Input: dimensioned drawing with shaded views. Units: mm. Origin: part minimum x, y, z. A direction names the side the tool comes from. Round coordinates to 2 decimals unless told otherwise and drop trailing zeros. Order: outer loops, then holes, each group sorted by start corner. A loop starts at its lowest first (then second) coordinate and runs counter-clockwise, first axis right, second up. Notation, with made-up numbers: M -30,1 L 5,1 A21 ccw 5,31 Z; hole C 4,8.5 d9. An arc over 180 degrees is marked long. Use one line per item in the form item = value. Start each with the question number.
Q1. Contact query for flat-ended pins moving along their axis: pin 1 (9 mm diameter, centred on x = 22, z = 10, fed in from +Y); pin 2 (1 mm diameter, centred on x = 29, z = 6, fed in from -Y); pin 3 (1.2 mm diameter, centred on x = 14, y = 1, fed in from -Z). Output: stop coordinate, or through.
Q2. Reachability of the marked faces 4, 5 and 6 from +Z, -Z, +X, -X, +Y, -Y: full face, straight path, thin tool, end or side. Return the list, or none.
Q3. Section C-C (z = 3.75). Return the cut outline in (x, y), plus the area to 3 significant figures.
Q4. Section D-D (x = 9.5). Return the cut outline in (y, z).
Q5. Pull-direction query (X, two-part tool) for the marked faces 1, 2 and 3; classes: pulls with the +X half, pulls with the -X half, needs draft (parallel to the pull), parting line crosses it, or undercut.
Q6. Section B-B (x = 22). Return the cut outline in (y, z).
Q7. Material intervals for probe 1 along X at (y, z) = (21.75, 10); probe 2 along X at (y, z) = (4.05, 10); probe 3 along Y at (x, z) = (31, 2), sorted ascending.
Q8. Section A-A (y = 14.5). Return the cut outline in (x, z).
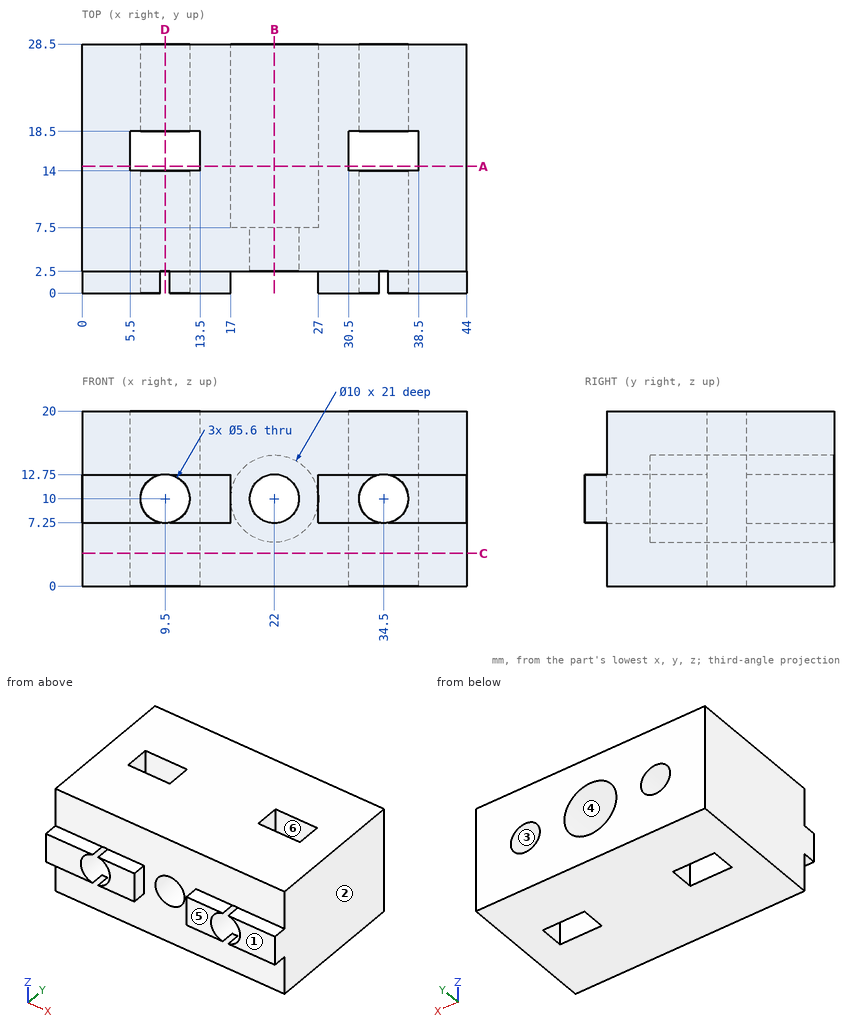
Results list:
q1.pin_1 = 7.5
q1.pin_2 = 2.5
q1.pin_3 = 7.25
q2.face_4 = +Y
q2.face_5 = +Z, -Z, +X, -X, -Y
q2.face_6 = +Z, -Z
q3.outline = M 0,2.5 L 44,2.5 L 44,28.5 L 0,28.5 Z; hole M 5.5,14 L 13.5,14 L 13.5,18.5 L 5.5,18.5 Z; hole M 30.5,14 L 38.5,14 L 38.5,18.5 L 30.5,18.5 Z
q3.area = 1,070 mm2
q4.outline = M 2.5,0 L 14,0 L 14,7.2 L 2.5,7.2 Z; M 2.5,12.8 L 14,12.8 L 14,20 L 2.5,20 Z; M 18.5,0 L 28.5,0 L 28.5,7.2 L 18.5,7.2 Z; M 18.5,12.8 L 28.5,12.8 L 28.5,20 L 18.5,20 Z
q5.face_1 = needs draft
q5.face_2 = pulls with the +X half
q5.face_3 = undercut
q6.outline = M 2.5,0 L 28.5,0 L 28.5,5 L 7.5,5 L 7.5,7.2 L 2.5,7.2 Z; M 2.5,12.8 L 7.5,12.8 L 7.5,15 L 28.5,15 L 28.5,20 L 2.5,20 Z
q7.probe_1 = 0 to 6.7, 12.3 to 17, 27 to 31.7, 37.3 to 44
q7.probe_2 = 0 to 6.7, 12.3 to 19.2, 24.8 to 31.7, 37.3 to 44
q7.probe_3 = 2.5 to 14, 18.5 to 28.5
q8.outline = M 0,0 L 5.5,0 L 5.5,20 L 0,20 Z; M 13.5,0 L 30.5,0 L 30.5,20 L 13.5,20 Z; M 38.5,0 L 44,0 L 44,20 L 38.5,20 Z; hole C 22,10 d10
